```python
from build123d import *

# Parameters (mm, degrees)
F3_DEPTH  = 177.8
F4_R      = 7.62
F5_DEPTH  = 19.05
F6_SIZE2  = 18.860161823
F6_SIZE   = 7.62
F4_R_2    = 5.715
F7_DEPTH  = 5.08
F8_R      = 5.07999
F9_R      = 6.35
F10_DEPTH = 50.8
F11_SCALE = 0.85684223


# Not quite as in the source:
# - a fillet or chamfer is up to 0.001 mm smaller than in the source, because OpenCascade refuses the exact size


with BuildPart() as f1:
    # F0 (on Front) → F1 (revolve)
    with BuildSketch(Plane.XZ):
        with BuildLine():
            Line((-38.2711647941, 0), (0, 0))
            Line((0, 0), (0, 146.0500033258))
            Line((0, 146.0500033258), (0, 152.4))
            ThreePointArc((0, 152.4), (-33.2006597867, 137.6319951518), (-44.4655865431, 103.0852268133))
            add(Edge.make_bspline(
                [(-44.4655865431, 0), (-47.1114422222, 11.762074058), (-53.3469479224, 35.8297600734), (-37.8272166921, 76.0482431769), (-42.543614325, 94.8604386904), (-44.4655865431, 103.0852268133)],
                knots=[0, 0, 0, 0, 0.3424224234, 0.7066775859, 1, 1, 1, 1], degree=3))
            Line((-44.4655865431, 0), (-38.2711647941, 0))
        make_face()
    revolve(axis=Axis((0, 0, 76.2), (0, 0, 1)))

    # F2 (on Top) → F3 (cut)
    with BuildSketch(Plane.XY):
        Polygon((25.6092443837, -36.641700535), (-25.1907556163, -36.641700535), (-46.7807556163, -36.641700535), (-46.7807556163, -67.121700535), (42.1192443837, -67.121700535), (42.1192443837, -36.641700535), align=None)
    extrude(amount=F3_DEPTH, mode=Mode.SUBTRACT)

    # F4 (on face) → F5 (join)
    with BuildSketch(Plane.XZ.offset(36.641700535)):
        with Locations((0, 97.9992443837)):
            Circle(F4_R)
    extrude(amount=F5_DEPTH)

    # F6
    f6_edges = [f1.edges().sort_by_distance(p)[0] for p in [
        (-7.62, -55.691701, 97.999244),
    ]]
    f6_side = f1.faces().sort_by_distance((0, -55.691701, 97.999244))[0]
    chamfer(f6_edges, length=F6_SIZE, length2=F6_SIZE2, reference=f6_side)

    # F4 (on face) → F7 (join)
    with BuildSketch(Plane.XZ.offset(36.641700535)):
        with Locations((-12.7, 112.2232443837)):
            Circle(F4_R_2)
        with Locations((12.7, 112.2232443837)):
            Circle(F4_R_2)
    extrude(amount=F7_DEPTH)

    # F8 (radius 5.08 in the source; OpenCascade refuses exactly that, so slightly less here)
    f8_edges = [f1.edges().sort_by_distance(p)[0] for p in [
        (-18.415, -41.721701, 112.223244),
        (6.985, -41.721701, 112.223244),
    ]]
    fillet(f8_edges, radius=F8_R)

    # F9 (on face) → F10 (cut)
    with BuildSketch(Plane(origin=(0, 0, 0), x_dir=(1, 0, 0), z_dir=(0, 0, -1))):
        Circle(F9_R)
    extrude(amount=-F10_DEPTH, mode=Mode.SUBTRACT)


with BuildPart() as f1_1:
    # F11: moved
    add(f1.part.scale(F11_SCALE))


solid = f1_1.part
```
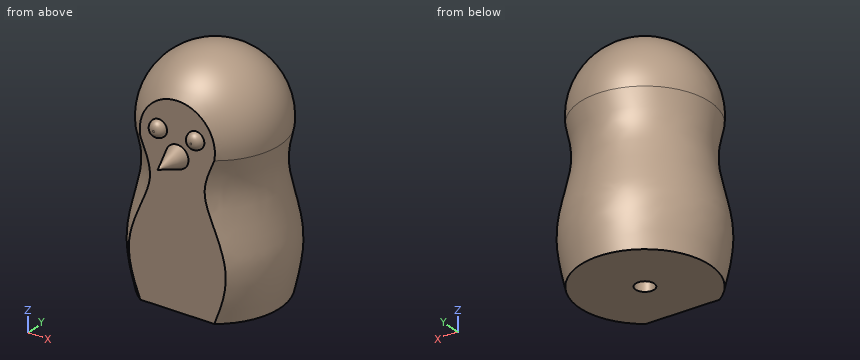
Input: part model. Units: mm. Frame: model coordinates. Coordinates: 2 decimals unless noted, no trailing zeros. Write each loop counter-clockwise with the first axis right and the second up, starting at its lowest first coordinate (ties: lowest second). Pieces come first, ordered by that corner, then holes. Notation, with made-up numbers: (9, -7) -> (64, -7) arc R20 cw to (64, 31) -> close; hole circle Ø6 at (-1, 18.25). An arc over 180 degrees is marked (long way). Write each question's results on one line, items separated by ' | '.
Item 1: Pin query (flat end, axial travel): pin 1 Ø10 at (y, z) = (-34.5, 23) entering from -X; pin 2 Ø1.5 at (y, z) = (31, 48) entering from -X; pin 3 Ø1 at (x, z) = (25.5, 22.5) entering from -Y. Return the tip coordinate at first contact, or that it passes through.
Conclusion:
pin 1: stops at x = -30.12 | pin 2: stops at x = -24.49 | pin 3: stops at y = -31.4
Item 2: Section query A-A on z = 112. Return loops of the section in (x, y), plus the area to 3 significant figures.
Conclusion:
outline: (-9.62, -31.4) -> (9.62, -31.4) arc R32.84 ccw (long way) to start | area: 3,370 mm^2
Item 3: Material intervals for probe 1 along Y at (x, z) = (0, 29); probe 2 along Z at (x, y) = (-31.5, -1); probe 3 along Y at (x, z) = (0, 12.5), sorted ascending.
Conclusion:
probe 1: y = -31.4 to -5.44, 5.44 to 42.2 | probe 2: z = 0 to 114.05 | probe 3: y = -31.4 to -5.44, 5.44 to 40.81
